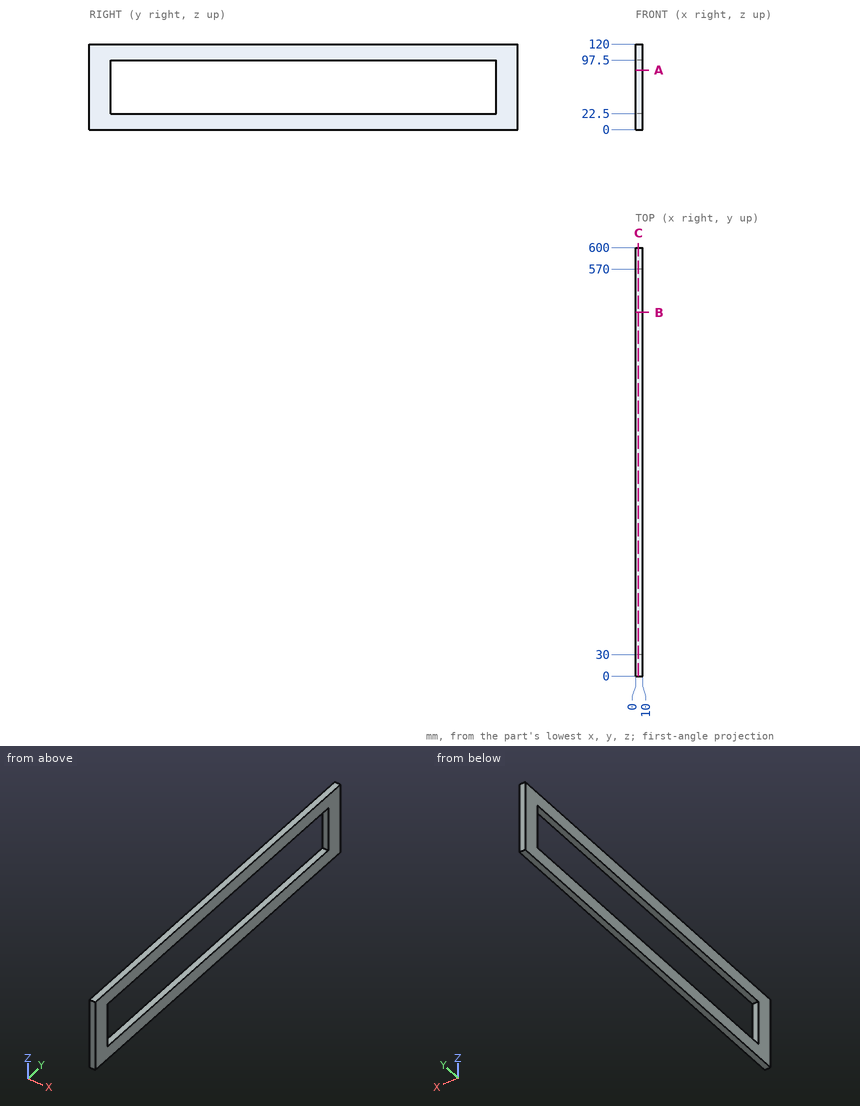
Geometry check sheet. Reference: drawing and pictorial views, mm from the part's lowest x, y, z. Coordinates: 2 decimals unless noted, no trailing zeros. Write each loop counter-clockwise with the first axis right and the second up, starting at its lowest first coordinate (ties: lowest second). Pieces come first, ordered by that corner, then holes. Notation, with made-up numbers: (-31.75, -33.75) -> (20.25, -33.75) arc R17 ccw to (20.25, -5.75) -> close; hole circle Ø5 at (-38, 34). An arc over 180 degrees is marked (long way). Use a Markdown table: item, result.
1. Scan lines: line 1 along Y through (x, z) = (5.5, 80.5); line 2 along Z through (x, y) = (6, 449). Record each from-to range of solid material in increasing order.
Reported:
| item | result |
|---|---|
| line 1 | y = 0 to 30, 570 to 600 |
| line 2 | z = 0 to 22.5, 97.5 to 120 |
2. Sectioned sample at A-A (z = 83.5). Enter the section's corners in (x, y).
Reported:
| item | result |
|---|---|
| outline | (0, 0) -> (10, 0) -> (10, 30) -> (0, 30) -> close; (0, 570) -> (10, 570) -> (10, 600) -> (0, 600) -> close |
3. Sectioned sample at C-C (x = 3.75). Enter the section's corners in (y, z), plus the area to 3 significant figures.
Reported:
| item | result |
|---|---|
| outline | (0, 0) -> (600, 0) -> (600, 120) -> (0, 120) -> close; hole (30, 22.5) -> (570, 22.5) -> (570, 97.5) -> (30, 97.5) -> close |
| area | 31,500 mm2 |
4. Sectioned sample at B-B (y = 509.5). Enter the section's corners in (x, z), plus the area to 3 significant figures.
Reported:
| item | result |
|---|---|
| outline | (0, 0) -> (10, 0) -> (10, 22.5) -> (0, 22.5) -> close; (0, 97.5) -> (10, 97.5) -> (10, 120) -> (0, 120) -> close |
| area | 450 mm2 |
